Could you check a few things on this model? Use its own coordinates, in mm. A direction names the side the tool comes from. Coordinates: 2 decimals unless noted, no trailing zeros. Loops run counter-clockwise (first coordinate to the right, second up) from the corner with the lowest first, then second, coordinate; pieces in that order, holes last. Notation, with made-up numbers: (78, 86.5) -> (99, 86.5) arc R29 cw to (99, 110.5) -> close; hole circle Ø6 at (50.5, -40). An arc over 180 degrees is marked (long way). One line per question, with ' | ' between items.
from build123d import *

# Parameters (mm, degrees)
ESBO_O3_W                = 47.4
ESBO_O3_H                = 47.4
RESSALTO_EXTRUS_O2_DEPTH = 1.6
ESBO_O5_W                = 51
ESBO_O5_H                = 51
RESSALTO_EXTRUS_O3_DEPTH = 1.6
CORTE_EXTRUS_O1_DEPTH    = 3.2
ESBO_O7_W                = 8
ESBO_O7_H                = 3.6
RESSALTO_EXTRUS_O4_DEPTH = 8
FILETE1_R                = 1
ESBO_O8_W                = 51
ESBO_O8_H                = 51
RESSALTO_EXTRUS_O5_DEPTH = 3.2
ESBO_O9_W                = 34.8
ESBO_O9_H                = 10.8
CORTE_EXTRUS_O2_DEPTH    = 3.2
ESBO_O10_R               = 1.6
CORTE_EXTRUS_O3_DEPTH    = 37.939139135
ESBO_O11_R               = 1.8
CORTE_EXTRUS_O4_DEPTH    = 2.4
ESBO_O11_2_R             = 1.8
CORTE_EXTRUS_O5_DEPTH    = 54.120335089


with BuildPart() as part:
    # Esboço3 → Ressalto-extrusão2 (new body)
    with BuildSketch(Plane.XY):
        Rectangle(ESBO_O3_W, ESBO_O3_H)
    extrude(amount=RESSALTO_EXTRUS_O2_DEPTH)

    # Esboço5 → Ressalto-extrusão3 (add)
    with BuildSketch(Plane(origin=(0, 0, 0), x_dir=(-1, 0, 0), z_dir=(0, 0, -1))):
        Rectangle(ESBO_O5_W, ESBO_O5_H)
    extrude(amount=RESSALTO_EXTRUS_O3_DEPTH)

    # Esboço6 → Corte-extrusão1 (cut)
    with BuildSketch(Plane(origin=(0, 0, -1.6), x_dir=(-1, 0, 0), z_dir=(0, 0, -1))):
        Polygon((3.535533906, 0), (20, 16.464466094), (20, -16.464466094), align=None)
        Polygon((-16.464466094, -20), (0, -3.535533906), (16.464466094, -20), align=None)
        Polygon((-20, 16.464466094), (-3.535533906, 0), (-20, -16.464466094), align=None)
        Polygon((-16.464466094, 20), (0, 3.535533906), (16.464466094, 20), align=None)
    extrude(amount=-CORTE_EXTRUS_O1_DEPTH, mode=Mode.SUBTRACT)

    # Esboço7 → Ressalto-extrusão4 (add)
    with BuildSketch(Plane.XY.offset(1.6)):
        Polygon((-23.7, 16.1), (-23.7, -7.1), (-20.1, -7.1), (-20.1, -5.1), (-23, -5.1), (-23, -3.1), (-20.1, -3.1), (-20.1, 1.3), (-23, 1.3), (-23, 3.3), (-20.1, 3.3), (-20.1, 12.1), (-23, 12.1), (-23, 14.1), (-21.7, 14.1), (-21.7, 16.1), align=None)
        with Locations((-19.7, 21.9)):
            Rectangle(ESBO_O7_W, ESBO_O7_H)
    ressalto_extrus_o4 = extrude(amount=RESSALTO_EXTRUS_O4_DEPTH)

    # Espelhar1: Ressalto-extrusão4 across plane
    add(ressalto_extrus_o4.mirror(Plane(origin=(0, 0, 0), x_dir=(0, 0, 1), z_dir=(1, 0, 0))))

    # Filete1
    # the kernel refuses this fillet: 1 mm, written as the material it takes off along each edge
    with BuildSketch(Plane(origin=(-23, 1.3, 9.6), x_dir=(-1, 0, 0), z_dir=(0, 1, 0)), Plane(origin=(-23, 12.1, 9.6), x_dir=(-1, 0, 0), z_dir=(0, 1, 0)), Plane(origin=(-23, -5.1, 9.6), x_dir=(-1, 0, 0), z_dir=(0, 1, 0))) as filete1_piece_1:
        with BuildLine():
            CenterArc((FILETE1_R, -FILETE1_R), FILETE1_R, 90, 90)
            Line((0, -FILETE1_R), (0, 0))
            Line((0, 0), (FILETE1_R, 0))
        make_face()
    extrude(amount=2, mode=Mode.SUBTRACT)
    with BuildSketch(Plane(origin=(23, 12.1, 9.6), x_dir=(1, 0, 0), z_dir=(0, 1, 0)), Plane(origin=(23, 1.3, 9.6), x_dir=(1, 0, 0), z_dir=(0, 1, 0)), Plane(origin=(23, -5.1, 9.6), x_dir=(1, 0, 0), z_dir=(0, 1, 0))) as filete1_piece_2:
        with BuildLine():
            CenterArc((FILETE1_R, FILETE1_R), FILETE1_R, 180, 90)
            Line((0, FILETE1_R), (0, 0))
            Line((0, 0), (FILETE1_R, 0))
        make_face()
    extrude(amount=2, mode=Mode.SUBTRACT)

    # Esboço8 → Ressalto-extrusão5 (add)
    with BuildSketch(Plane(origin=(0, 0, -1.6), x_dir=(-1, 0, 0), z_dir=(0, 0, -1))):
        Rectangle(ESBO_O8_W, ESBO_O8_H)
        Polygon((-16.464466094, -20), (16.464466094, -20), (0, -3.535533906), align=None, mode=Mode.SUBTRACT)
        Polygon((-20, -16.464466094), (-3.535533906, 0), (-20, 16.464466094), align=None, mode=Mode.SUBTRACT)
        Polygon((3.535533906, 0), (20, -16.464466094), (20, 16.464466094), align=None, mode=Mode.SUBTRACT)
        Polygon((0, 3.535533906), (16.464466094, 20), (-16.464466094, 20), align=None, mode=Mode.SUBTRACT)
    extrude(amount=RESSALTO_EXTRUS_O5_DEPTH)

    # Esboço9 → Corte-extrusão2 (cut)
    with BuildSketch(Plane.XY.offset(1.6)):
        with Locations((0, -18.3)):
            Rectangle(ESBO_O9_W, ESBO_O9_H)
    extrude(amount=-CORTE_EXTRUS_O2_DEPTH, mode=Mode.SUBTRACT)

    # Esboço10 → Corte-extrusão3 (cut, through all)
    with BuildSketch(Plane.XY.offset(1.6)):
        with Locations((7, -6.7)):
            Circle(ESBO_O10_R)
    extrude(amount=-CORTE_EXTRUS_O3_DEPTH, mode=Mode.SUBTRACT)

    # Esboço11 → Corte-extrusão4 (cut)
    with BuildSketch(Plane.XZ.offset(-20.1)):
        Polygon((-19.7, 8.833161507), (-22.5, 7.216580754), (-22.5, 3.983419246), (-19.7, 2.366838493), (-16.9, 3.983419246), (-16.9, 7.216580754), align=None)
        with Locations(Location((-19.7, 5.6, 0), (0, 0, 270))):
            Circle(ESBO_O11_R, mode=Mode.SUBTRACT)
    corte_extrus_o4 = extrude(amount=-CORTE_EXTRUS_O4_DEPTH, mode=Mode.SUBTRACT)

    # Esboço11<2> → Corte-extrusão5 (cut, through all)
    with BuildSketch(Plane.XZ.offset(-20.1)):
        with Locations(Location((-19.7, 5.6, 0), (0, 0, 270))):
            Circle(ESBO_O11_2_R)
    corte_extrus_o5 = extrude(amount=-CORTE_EXTRUS_O5_DEPTH, mode=Mode.SUBTRACT)

    # Espelhar2: Corte-extrusão4, Corte-extrusão5 across plane
    add(corte_extrus_o4.mirror(Plane(origin=(0, 0, 0), x_dir=(0, 0, 1), z_dir=(1, 0, 0))), mode=Mode.SUBTRACT)
    add(corte_extrus_o5.mirror(Plane(origin=(0, 0, 0), x_dir=(0, 0, 1), z_dir=(1, 0, 0))), mode=Mode.SUBTRACT)


solid = part.part
1) If we section it at C-C on y = 5: Please give me the cut outline in (x, z), and give its area (3 significant figures).
Data:
outline: (-25.5, -4.8) -> (-20, -4.8) -> (-20, 1.6) -> (-20.1, 1.6) -> (-20.1, 9.6) -> (-23.7, 9.6) -> (-23.7, 0) -> (-25.5, 0) -> close; (-8.54, -4.8) -> (-1.46, -4.8) -> (-1.46, 1.6) -> (-8.54, 1.6) -> close; (1.46, -4.8) -> (8.54, -4.8) -> (8.54, 1.6) -> (1.46, 1.6) -> close; (20, -4.8) -> (25.5, -4.8) -> (25.5, 0) -> (23.7, 0) -> (23.7, 9.6) -> (20.1, 9.6) -> (20.1, 1.6) -> (20, 1.6) -> close | area: 213 mm²
2) If we section it at B-B on y = 18.5: Please give me the cut outline in (x, z).
Data:
outline: (-25.5, -4.8) -> (-14.96, -4.8) -> (-14.96, 1.6) -> (-23.7, 1.6) -> (-23.7, 0) -> (-25.5, 0) -> close; (14.96, -4.8) -> (25.5, -4.8) -> (25.5, 0) -> (23.7, 0) -> (23.7, 1.6) -> (14.96, 1.6) -> close
3) If we section it at A-A on x = 7: Please give me the cut outline in (y, z).
Data:
outline: (-25.5, -4.8) -> (-20, -4.8) -> (-20, -1.6) -> (-23.7, -1.6) -> (-23.7, 0) -> (-25.5, 0) -> close; (-10.54, -4.8) -> (-8.3, -4.8) -> (-8.3, 1.6) -> (-10.54, 1.6) -> close; (-5.1, -4.8) -> (-3.46, -4.8) -> (-3.46, 1.6) -> (-5.1, 1.6) -> close; (3.46, -4.8) -> (10.54, -4.8) -> (10.54, 1.6) -> (3.46, 1.6) -> close; (20, -4.8) -> (25.5, -4.8) -> (25.5, 0) -> (23.7, 0) -> (23.7, 1.6) -> (20, 1.6) -> close
4) If we section it at D-D on x = -1.5: Please give me the cut outline in (y, z), and give its area (3 significant figures).
Data:
outline: (-25.5, -4.8) -> (-20, -4.8) -> (-20, -1.6) -> (-23.7, -1.6) -> (-23.7, 0) -> (-25.5, 0) -> close; (-5.04, -4.8) -> (5.04, -4.8) -> (5.04, 1.6) -> (-5.04, 1.6) -> close; (20, -4.8) -> (25.5, -4.8) -> (25.5, 0) -> (23.7, 0) -> (23.7, 1.6) -> (20, 1.6) -> close | area: 117 mm²
5) On a 3-axis mill with a long thin cutter (end or side, diameter ignored), from which of +Z, -Z, +X, -X, +Y, -Y can I reach the whole of each face in a straight line? I mean faces 4 (the face through (-22, -7.1, 6)), 5 (the face through (-21.08, 21.283, 8.036)), 6 (the face through (16.9, 21, 6)), 7 (the face through (-22, -3.1, 6)). Say none if no direction works.
Data:
face 4: +Z, +X, -X, -Y | face 5: none | face 6: -Y | face 7: +Z
6) I'm going to push flat-ended pins straight in: pin 1 Ø6 at (x, z) = (7, 2) entering from +Y; pin 2 Ø3 at (x, z) = (22, 4.5) entering from -Y; pin 3 Ø2.5 at (x, z) = (-18, 5.5) entering from -Y; pin 4 Ø2 at (y, z) = (2, 7) entering from -X. Where does each tip first touch, or does it pass through?
Data:
pin 1: y = 25.5 | pin 2: y = -7.1 | pin 3: y = 20.1 | pin 4: x = -23.7
7) I need wall thicknesses on line 1 along X through (y, z) = (23.25, 5.6); line 2 along Y through (x, z) = (-21, 3.75); line 3 along Y through (x, z) = (22, 5.75). Which ranges of each line are inside material? Lowest first, please. Write a range as from..to.
Data:
line 1: -23.7..-21.5, -17.9..-15.7, 15.7..17.9, 21.5..23.7 | line 2: -7.1..-5.1, -3.1..1.3, 3.3..12.1, 22.5..23.7 | line 3: -7.1..-5.1, -3.1..1.3, 3.3..12.1, 14.1..16.1, 22.5..23.7
8) We'd pull the mould along X, two halves only. Please class faces 1 (the face through (22, 3.3, 6)), 2 (the face through (-21, -23.7, 1)), 3 (the face through (-23.7, 5, 5)): pulls with the +X half, pulls with the -X half, needs draft (parallel to the pull), parting line crosses it, or undercut.
Data:
face 1: undercut | face 2: needs draft | face 3: pulls with the -X half
